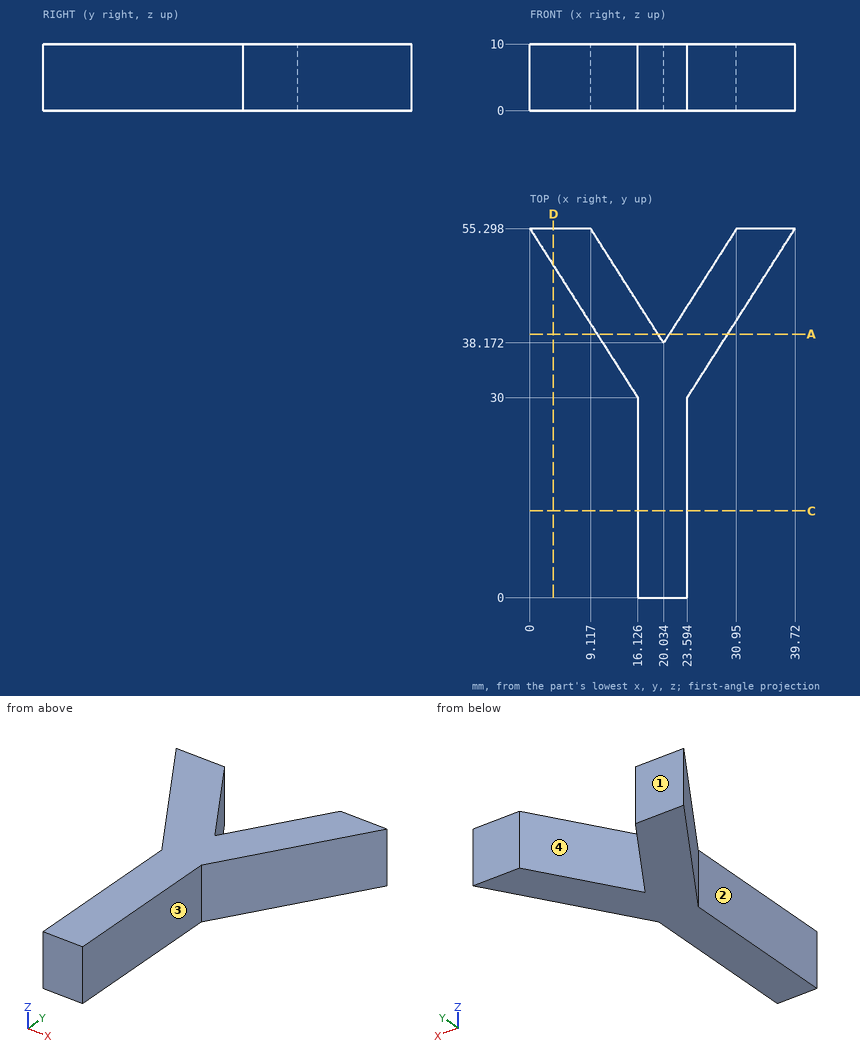
Verification items for this drawing (mm, ordinates from the low corner). Give positions to 0.01 mm unless a question says otherwise; leave off trailing zeros. Loops run counter-clockwise (first coordinate to the right, second up) from the corner with the lowest first, then second, coordinate; pieces in that order, holes last. Notation, with made-up numbers: M 32.25,76.25 L 56.25,76.25 A17 cw 56.25,84.25 Z; hole C 47.25,79.25 d3. An arc over 180 degrees is marked long. Answer as a JSON object with one key per item and string values. Group by question number.
Q1. Material ranges on line 1 along X through (y, z) = (17, 1.25) (1 decimal); line 2 along X through (y, z) = (50, 8) (1 decimal); line 3 along X through (y, z) = (41, 4.25) (1 decimal), recorded low to high. Write a range as [from, to].
Q2. Cross-section at A-A on y = 39.5. Record the cut outline in (x, z).
Q3. Go/stop test with flat-tipped pins: P1, Ø3, axis at y = 21.5, z = 6, coming from the +X side; P2, Ø3, axis at y = 10.5, z = 3.5, coming from the -X side. Record where each tip stops, or that it passes through.
Q4. Cross-section at D-D on x = 3.5. Record the cut outline in (y, z), then the cut area to 3 significant figures.
Q5. Cross-section at C-C on y = 13. Record the cut outline in (x, z) (1 decimal).
Q6. Release check for a two-part mould opening along X. For the marked faces 1, 2, 3 and 4 record: released by +X, released by -X, zero draft, split by the parting line, or undercut.
Evaluation:
{
 "1": {"line 1": "x = [16.1, 23.6]", "line 2": "x = [3.4, 12.5], [27.6, 36.3]", "line 3": "x = [9.1, 18.2], [21.8, 30.6]"},
 "2": {"outline": "M 10.07,0 L 19.19,0 L 19.19,10 L 10.07,10 Z; M 20.88,0 L 29.65,0 L 29.65,10 L 20.88,10 Z"},
 "3": {"P1": "stops at x = 23.59", "P2": "stops at x = 16.13"},
 "4": {"outline": "M 49.81,0 L 55.3,0 L 55.3,10 L 49.81,10 Z", "area": "54.9 mm2"},
 "5": {"outline": "M 16.1,0 L 23.6,0 L 23.6,10 L 16.1,10 Z"},
 "6": {"face 1": "zero draft", "face 2": "released by -X", "face 3": "released by +X", "face 4": "undercut"}
}
